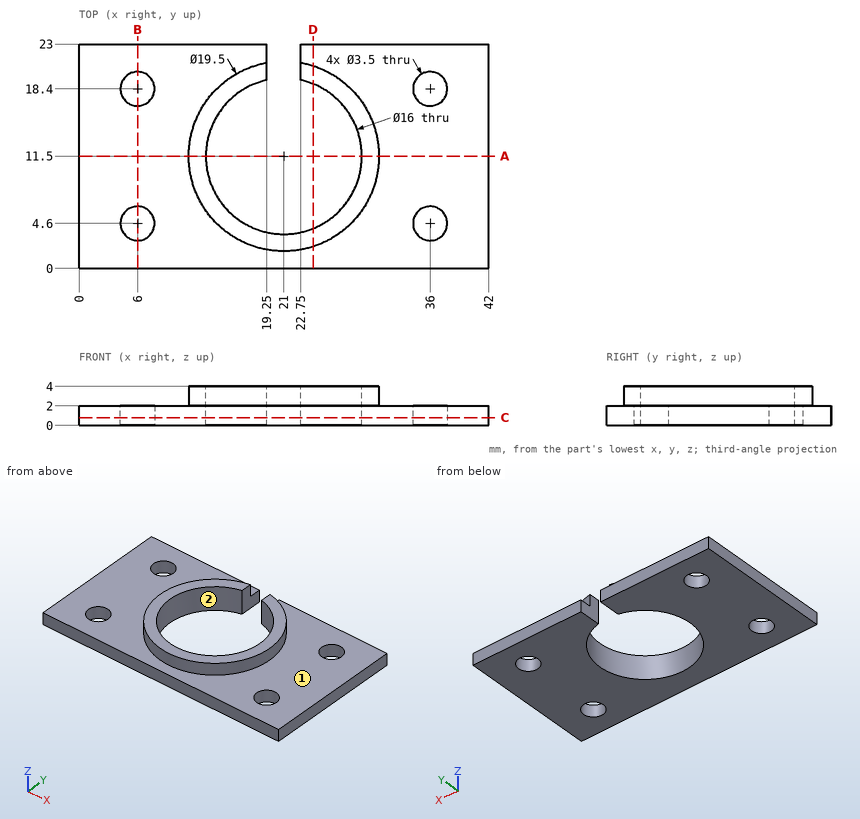
Check sheet for the drawn part. Datum: minimum x, y, z corner. Units: mm. Round coordinates to 2 decimals unless told otherwise and drop trailing zeros. Write each loop counter-clockwise with the first axis right and the second up, starting at its lowest first coordinate (ties: lowest second). Pieces come first, ordered by that corner, then holes. Notation, with made-up numbers: (18.25, 61) -> (65.25, 61) arc R21 ccw to (65.25, 90) -> close; hole circle Ø7 at (10.25, 57.5). An arc over 180 degrees is marked (long way). Put each result on its own line as item: value.
(1) Material ranges on line 1 (Y direction, x = 36, z = 1.05); line 2 (X direction, y = 19.75, z = 0.4); line 3 (X direction, y = 11.5, z = 2.8), recorded low to high.
Values found:
line 1: y = 0 to 2.85, 6.35 to 16.65, 20.15 to 23
line 2: x = 0 to 4.89, 7.11 to 19.25, 22.75 to 34.89, 37.11 to 42
line 3: x = 11.25 to 13, 29 to 30.75
(2) Go/stop test with a flat-tipped pin: pin 1 Ø4.5 at (x, y) = (6, 18.4) entering from +Z. Record where the tip stops, or that it passes through.
Values found:
pin 1: stops at z = 2
(3) Sectioned sample at A-A (y = 11.5). Enter the section's corners in (x, z).
Values found:
outline: (0, 0) -> (13, 0) -> (13, 4) -> (11.25, 4) -> (11.25, 2) -> (0, 2) -> close; (29, 0) -> (42, 0) -> (42, 2) -> (30.75, 2) -> (30.75, 4) -> (29, 4) -> close
(4) Mould release check, pull along Y, two halves, no side actions. Record for the marked faces 1 and 2: released by +Y, released by -Y, zero draft, split by the parting line, or undercut.
Values found:
face 1: zero draft
face 2: undercut
(5) Sectioned sample at D-D (x = 24). Enter the section's corners in (y, z), plus the area to 3 significant figures.
Values found:
outline: (0, 0) -> (4.08, 0) -> (4.08, 4) -> (2.22, 4) -> (2.22, 2) -> (0, 2) -> close; (18.92, 0) -> (23, 0) -> (23, 2) -> (20.78, 2) -> (20.78, 4) -> (18.92, 4) -> close
area: 23.8 mm^2
(6) Sectioned sample at B-B (x = 6). Enter the section's corners in (y, z).
Values found:
outline: (0, 0) -> (2.85, 0) -> (2.85, 2) -> (0, 2) -> close; (6.35, 0) -> (16.65, 0) -> (16.65, 2) -> (6.35, 2) -> close; (20.15, 0) -> (23, 0) -> (23, 2) -> (20.15, 2) -> close
(7) Sectioned sample at C-C (z = 0.8). Enter the section's corners in (x, y), plus the area to 3 significant figures.
Values found:
outline: (0, 0) -> (42, 0) -> (42, 23) -> (22.75, 23) -> (22.75, 19.31) arc R8 cw (long way) to (19.25, 19.31) -> (19.25, 23) -> (0, 23) -> close; hole circle Ø3.5 at (6, 4.6); hole circle Ø3.5 at (6, 18.4); hole circle Ø3.5 at (36, 4.6); hole circle Ø3.5 at (36, 18.4)
area: 714 mm^2
